Here's how the part is built. I have some questions about the finished solid (model axes, mm). Give positions to 0.01 mm unless a question says otherwise; leave off trailing zeros. Order: outer loops, then holes, each group sorted by start corner. A loop starts at its lowest first (then second) coordinate and runs counter-clockwise, first axis right, second up.
from build123d import *

# Parameters (mm, degrees)
SKETCH1_W           = 95
SKETCH1_H           = 30
BOSS_EXTRUDE1_DEPTH = 3
SKETCH4_W           = 3
SKETCH4_H           = 5
BOSS_EXTRUDE2_DEPTH = 3
SKETCH5_W           = 3
SKETCH5_H           = 39
BOSS_EXTRUDE3_DEPTH = 15
SKETCH2_R           = 3
CUT_EXTRUDE1_DEPTH  = 80.113842025
LPATTERN1_COUNT     = 3
LPATTERN1_PITCH     = 35
SKETCH6_W           = 2.95
SKETCH6_H           = 8.706192548
SKETCH6_W_2         = 22.8
SKETCH6_H_2         = 6.5
CUT_EXTRUDE2_DEPTH  = 80.113842025
FILLET3_R           = 5
FILLET4_R           = 1


with BuildPart() as part:
    # Sketch1 → Boss-Extrude1 (new body)
    with BuildSketch(Plane(origin=(0, 0, 0), x_dir=(0, 0, -1), z_dir=(1, 0, 0))):
        with Locations((17.5, 15)):
            Rectangle(SKETCH1_W, SKETCH1_H)
    extrude(amount=BOSS_EXTRUDE1_DEPTH)

    # Sketch4 → Boss-Extrude2 (add)
    with BuildSketch(Plane(origin=(0, 0, 0), x_dir=(1, 0, 0), z_dir=(0, 1, 0))):
        with Locations((1.5, -17.5)):
            Rectangle(SKETCH4_W, SKETCH4_H)
    boss_extrude2 = extrude(amount=-BOSS_EXTRUDE2_DEPTH)

    # Sketch5 → Boss-Extrude3 (add)
    with BuildSketch(Plane(origin=(0, 30, 0), x_dir=(1, 0, 0), z_dir=(0, 1, 0))):
        with Locations((1.5, -10.5)):
            Rectangle(SKETCH5_W, SKETCH5_H)
    extrude(amount=BOSS_EXTRUDE3_DEPTH)

    # Sketch2 → Cut-Extrude1 (cut, through all)
    with BuildSketch(Plane(origin=(3, 0, 0), x_dir=(0, 0, -1), z_dir=(1, 0, 0))):
        with Locations((28.2, 23.5)):
            Circle(SKETCH2_R)
        with Locations((-9.3, 35)):
            Circle(SKETCH2_R)
    extrude(amount=-CUT_EXTRUDE1_DEPTH, mode=Mode.SUBTRACT)

    # LPattern1: Boss-Extrude2 ×3
    with Locations(*[(0, 0, -i * LPATTERN1_PITCH) for i in range(1, LPATTERN1_COUNT)]):
        add(boss_extrude2)

    # Sketch6 → Cut-Extrude2 (cut, through all)
    with BuildSketch(Plane(origin=(3, 0, 0), x_dir=(0, 0, -1), z_dir=(1, 0, 0))):
        with Locations((12.746364518, 27.853096274)):
            Rectangle(SKETCH6_W, SKETCH6_H)
        with Locations((53.6, 26.75)):
            Rectangle(SKETCH6_W_2, SKETCH6_H_2)
    extrude(amount=-CUT_EXTRUDE2_DEPTH, mode=Mode.SUBTRACT)

    # Fillet3
    # the kernel refuses this fillet: 5 mm, written as the material it adds along each edge
    with BuildSketch(Plane(origin=(0, 30, -9), x_dir=(0, 1.1824837095993706e-12, -1.0), z_dir=(1, 0, 0))) as fillet3_piece_1:
        with BuildLine():
            CenterArc((5, 4.189814842), FILLET3_R, 180, 56.925635132)
            Line((0, 4.189814842), (0, 0))
            Line((0, 0), (2.271364518, 0))
        make_face()
    extrude(amount=3)
    # the kernel refuses this fillet: 5 mm, written as the material it takes off along each edge
    with BuildSketch(Plane(origin=(15.5, 45, 30), x_dir=(0, 0, -1), z_dir=(-1, 0, 0)), Plane(origin=(15.5, 23.5, -65), x_dir=(0, -1, 0), z_dir=(-1, 0, 0))) as fillet3_2_piece_1:
        with BuildLine():
            CenterArc((FILLET3_R, FILLET3_R), FILLET3_R, 180, 90)
            Line((0, FILLET3_R), (0, 0))
            Line((0, 0), (FILLET3_R, 0))
        make_face()
    extrude(amount=28, mode=Mode.SUBTRACT)
    with BuildSketch(Plane(origin=(-12.5, 45, -9), x_dir=(0, -1, 0), z_dir=(1, 0, 0))) as fillet3_2_piece_2:
        with BuildLine():
            CenterArc((FILLET3_R, -FILLET3_R), FILLET3_R, 90, 90)
            Line((0, -FILLET3_R), (0, 0))
            Line((0, 0), (FILLET3_R, 0))
        make_face()
    extrude(amount=28, mode=Mode.SUBTRACT)

    # Fillet4
    fillet4_edges = [part.edges().sort_by_distance(p)[0] for p in [
        (1.5, 30, -11.271364518),
        (1.5, 30, -14.221364518),
        (1.5, 30, -42.2),
    ]]
    fillet(fillet4_edges, radius=FILLET4_R)


solid = part.part
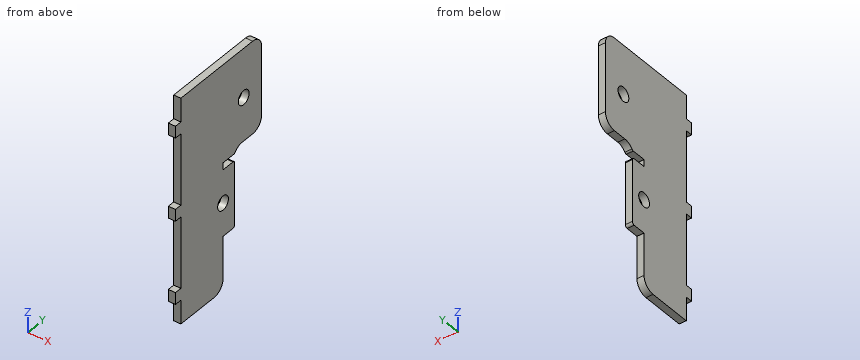
Q1. If we section it at B-B on y = 28: List the corners of the cut face in (x, z) for me, plus the area to 3 significant figures.
Filled sheet:
outline: (0, -42.2) - (3, -42.2) - (3, -14.22) - (0, -14.22) - close; (0, -11.27) - (3, -11.27) - (3, 30) - (0, 30) - close
area: 208 mm2
Q2. I'm going to push flat-ended pins straight in: P1, Ø1.5, axis at x = 1.5, y = -2, coming from the -Z side; P2, Ø7, axis at y = 23.5, z = -28.2, coming from the +X side; P3, Ø1, axis at x = 2, z = -32, coming from the +Y side; P4, Ø0.9, axis at x = 2, y = -2, coming from the +Z side. Where does each tip first touch, or does it pass through?
Filled sheet:
P1: stops at z = -55
P2: stops at x = 3
P3: stops at y = 30
P4: stops at z = 20
Q3. If we section it at C-C on z = 9.3: List the corners of the cut face in (x, y) for me, plus the area to 3 significant figures.
Filled sheet:
outline: (0, 0) - (3, 0) - (3, 32) - (0, 32) - close; (0, 38) - (3, 38) - (3, 45) - (0, 45) - close
area: 117 mm2
Q4. If we section it at D-D on z = -45.5: List the corners of the cut face in (x, y) for me, plus the area to 3 significant figures.
Filled sheet:
outline: (0, 0) - (3, 0) - (3, 23.5) - (0, 23.5) - close
area: 70.5 mm2
Q5. I need wall thicknesses on L1, parallel to Y at x = 0.85, z = -28.2; L2, parallel to Z at x = 2.55, y = 39; L3, parallel to Y at x = 1.35, z = -53.5. Which ranges of each line are inside material? Lowest first, please.
Filled sheet:
L1: y = 0 to 20.5, 26.5 to 30
L2: z = -9 to 30
L3: y = -3 to 23.5
Q6. If we section it at A-A on x = 2.15: Give the number of separate pieces and of enclosed holes in the cut face, plus the area to 3 significant figures.
Filled sheet:
separate pieces: 1
enclosed holes: 2
area: 3,240 mm2
